```python
from build123d import *

# Parameters (mm, degrees)
SKETCH1_R           = 9.625
SKETCH1_W           = 25
SKETCH1_H           = 20
BOSS_EXTRUDE1_DEPTH = 12
SKETCH2_R           = 2.25
CUT_EXTRUDE1_DEPTH  = 154.440542231


with BuildPart() as part:
    # Sketch1 → Boss-Extrude1 (new body)
    with BuildSketch(Plane(origin=(0, 0, 0), x_dir=(1, 0, 0), z_dir=(0, 1, 0))):
        with BuildLine():
            Line((-135, 15), (-39.3333, 15))
            Line((-39.3333, 15), (-39.3333, 10))
            Line((-39.3333, 10), (-48.3333, 10))
            Line((-48.3333, 10), (-48.3333, -10))
            Line((-48.3333, -10), (-39.3333, -10))
            Line((-39.3333, -10), (-39.3333, -15))
            Line((-39.3333, -15), (-135, -15))
            ThreePointArc((-135, -15), (-150, 0), (-135, 15))
        make_face()
        with Locations(Location((-135, 0, 0), (0, 0, 270))):
            Circle(SKETCH1_R, mode=Mode.SUBTRACT)
        with Locations((-107.5, 0)):
            Rectangle(SKETCH1_W, SKETCH1_H, mode=Mode.SUBTRACT)
        with Locations((-72.5, 0)):
            Rectangle(SKETCH1_W, SKETCH1_H, mode=Mode.SUBTRACT)
    extrude(amount=BOSS_EXTRUDE1_DEPTH)

    # Sketch2 → Cut-Extrude1 (cut, through all)
    with BuildSketch(Plane(origin=(0, 0, -15), x_dir=(-1, 0, 0), z_dir=(0, 0, -1))):
        with Locations((43.3333, 6)):
            Circle(SKETCH2_R)
    extrude(amount=-CUT_EXTRUDE1_DEPTH, mode=Mode.SUBTRACT)


solid = part.part
```
Build history of the part. All positions in model axes, mm. A direction names the side the tool comes from. Coordinates: 2 decimals unless noted, no trailing zeros. Write each loop counter-clockwise with the first axis right and the second up, starting at its lowest first coordinate (ties: lowest second). Pieces come first, ordered by that corner, then holes.
1. Band-saw the part on A-A, the plane x = -79.5. Give the cut face in (y, z).
Answer block:
outline: (0, -15) - (12, -15) - (12, -10) - (0, -10) - close; (0, 10) - (12, 10) - (12, 15) - (0, 15) - close
2. Pull direction Y, two halves, no side cores. Call faces 4 (the cylindrical face through (-45.48, 6.68, -12.54)), 5 (the flat face through (-120, 6, 0)), 6 (the flat face through (-94, 12, 0)): released by +Y, released by -Y, zero draft, split by the parting line, or undercut.
Answer block:
face 4: undercut
face 5: zero draft
face 6: released by +Y
3. 3-axis set-ups, long thin cutter, end or side, ignore diameter. For faces 1 (the flat face through (-39.333, 6, 12)), 2 (the flat face through (-73, 6, 10)), 3 (the flat face through (-46, 6, 10)): which of +Z, -Z, +X, -X, +Y, -Y reach the whole face in a straight line?
Answer block:
face 1: +Z, -Z, +X, +Y, -Y
face 2: +Y, -Y
face 3: +X, +Y, -Y
4. Drop a flat-ended pin along its axis: pin 1 (2 mm diameter, centred on y = 1.5, z = -5, fed in from -X). Give the stop position or say it passes through.
Answer block:
pin 1: stops at x = -149.46
5. Drill centre lines: probe 1 along X at (y, z) = (4, 0) (3 decimals); probe 2 along X at (y, z) = (1.75, -3.25); probe 3 along Z at (x, y) = (-77.5, 7.5). Where is each one in solid material? Low to high.
Answer block:
probe 1: x = -150 to -144.625, -125.375 to -120, -95 to -85, -60 to -48.333
probe 2: x = -149.64 to -144.06, -125.94 to -120, -95 to -85, -60 to -48.33
probe 3: z = -15 to -10, 10 to 15
6. Band-saw the part on D-D, the plane z = -8.5. Give the cut face in (x, y).
Answer block:
outline: (-147.36, 0) - (-139.52, 0) - (-139.52, 12) - (-147.36, 12) - close; (-130.48, 0) - (-120, 0) - (-120, 12) - (-130.48, 12) - close; (-95, 0) - (-85, 0) - (-85, 12) - (-95, 12) - close; (-60, 0) - (-48.33, 0) - (-48.33, 12) - (-60, 12) - close
7. Band-saw the part on B-B, the plane y = 6. Give the cut face in (x, z) (3 decimals).
Answer block:
outline: (-135, -15) - (-45.583, -15) - (-45.583, -10) - (-48.333, -10) - (-48.333, 10) - (-45.583, 10) - (-45.583, 15) - (-135, 15) arc R15 ccw to start; (-41.083, -15) - (-39.333, -15) - (-39.333, -10) - (-41.083, -10) - close; (-41.083, 10) - (-39.333, 10) - (-39.333, 15) - (-41.083, 15) - close; hole circle Ø19.25 at (-135, 0); hole (-120, -10) - (-95, -10) - (-95, 10) - (-120, 10) - close; hole (-85, -10) - (-60, -10) - (-60, 10) - (-85, 10) - close
8. Band-saw the part on C-C, the plane z = 0. Give the cut face in (x, y) (3 decimals).
Answer block:
outline: (-150, 0) - (-144.625, 0) - (-144.625, 12) - (-150, 12) - close; (-125.375, 0) - (-120, 0) - (-120, 12) - (-125.375, 12) - close; (-95, 0) - (-85, 0) - (-85, 12) - (-95, 12) - close; (-60, 0) - (-48.333, 0) - (-48.333, 12) - (-60, 12) - close
